The drawing under review shows one solid part. Ordinate dimensions are in mm from its lowest x, y, z. A direction names the side the tool comes from. Round coordinates to 2 decimals unless told otherwise and drop trailing zeros. Order: outer loops, then holes, each group sorted by start corner. A loop starts at its lowest first (then second) coordinate and runs counter-clockwise, first axis right, second up.
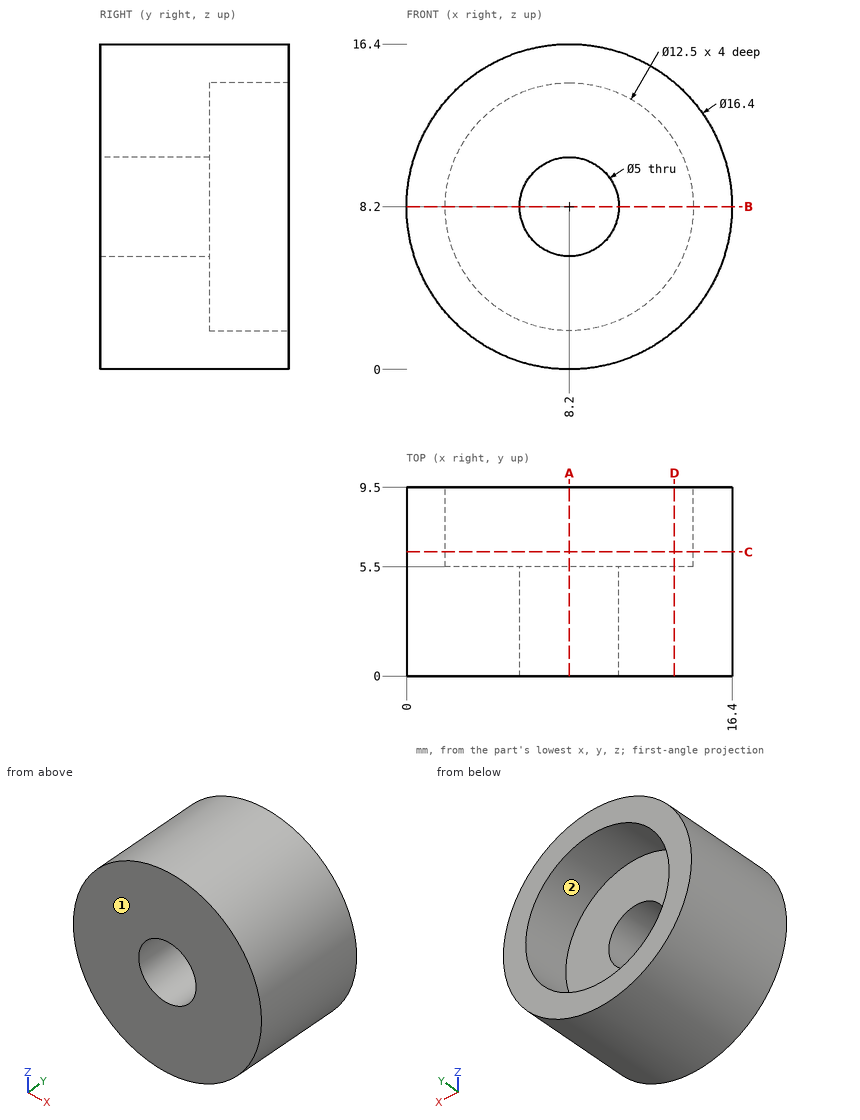
Q1. Clearance check with flat-ended pins moving along their axes: pin 1 (1 mm diameter, centred on x = 6, y = 4.5, fed in from +Z); pin 2 (2 mm diameter, centred on x = 7, z = 12.5, fed in from +Y); pin 3 (4 mm diameter, centred on y = 3.5, z = 11, fed in from -X). State where each tip first meets the part, or that it passes through.
Q2. Take a section at D-D, the plane x = 13.5. State the section outline as (y, z) points.
Q3. Take a section at B-B, the plane z = 8.2. State the section outline as (x, y) points.
Q4. Wall thickness on line 1 (X direction, y = 7.4, z = 8.2); line 2 (X direction, y = 3.3, z = 8.2); line 3 (Y direction, x = 11.75, z = 5.75): over which ranges is each line inside the solid? List them lowest first.
Q5. Take a section at C-C, the plane y = 6.25. State the section outline as (x, z) points, plus the area to 3 significant figures.
Q6. Take a section at A-A, the plane x = 8.2. State the section outline as (y, z) points.
Q7. Tool access review of the marked faces 1 and 2: name each direction out of +Z, -Z, +X, -X, +Y, -Y from which nothing blocks a thin tool from reaching the whole face with its end or side.
Working result:
1. pin 1: stops at z = 16.22
1. pin 2: stops at y = 5.5
1. pin 3: stops at x = 0.04
2. outline: (0, 1.94) - (9.5, 1.94) - (9.5, 4.89) - (5.5, 4.89) - (5.5, 11.51) - (9.5, 11.51) - (9.5, 14.46) - (0, 14.46) - close
3. outline: (0, 0) - (5.7, 0) - (5.7, 5.5) - (1.95, 5.5) - (1.95, 9.5) - (0, 9.5) - close; (10.7, 0) - (16.4, 0) - (16.4, 9.5) - (14.45, 9.5) - (14.45, 5.5) - (10.7, 5.5) - close
4. line 1: x = 0 to 1.95, 14.45 to 16.4
4. line 2: x = 0 to 5.7, 10.7 to 16.4
4. line 3: y = 0 to 5.5
5. outline: circle Ø16.4 at (8.2, 8.2); hole circle Ø12.5 at (8.2, 8.2)
5. area: 88.5 mm2
6. outline: (0, 0) - (9.5, 0) - (9.5, 1.95) - (5.5, 1.95) - (5.5, 5.7) - (0, 5.7) - close; (0, 10.7) - (5.5, 10.7) - (5.5, 14.45) - (9.5, 14.45) - (9.5, 16.4) - (0, 16.4) - close
7. face 1: +Z, -Z, +X, -X, -Y
7. face 2: +Y
